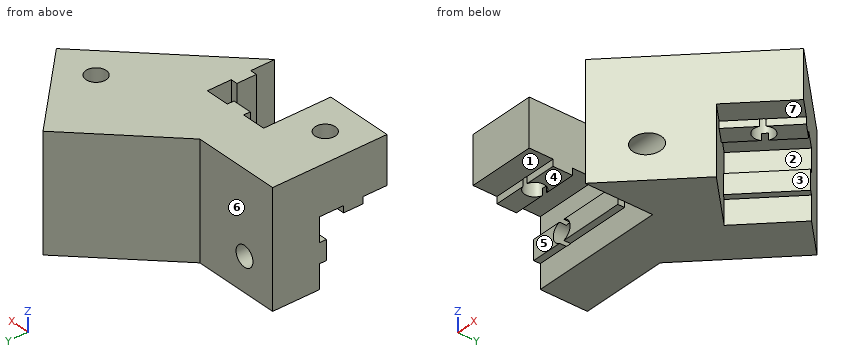
from build123d import *

# Parameters (mm, degrees)
MAIN_DEPTH          = 17
CUT_EXTRUDE1_DEPTH  = 10
SKETCH3_R           = 1.5
CUT_EXTRUDE2_DEPTH  = 18
SKETCH4_W           = 2.9
SKETCH4_H           = 1
SKETCH4_W_2         = 1
SKETCH4_H_2         = 2.9
BOSS_EXTRUDE1_DEPTH = 7
SKETCH5_W           = 15
SKETCH5_H           = 2.9
BOSS_EXTRUDE2_DEPTH = 1
SKETCH6_R           = 1.5
CUT_EXTRUDE3_DEPTH  = 18
BOSS_EXTRUDE3_DEPTH = 10
SKETCH8_R           = 1.5
CUT_EXTRUDE4_DEPTH  = 18
SKETCH9_R           = 1.5
CUT_EXTRUDE5_DEPTH  = 18.67766953


with BuildPart() as part:
    # Sketch1 → Main (new body)
    with BuildSketch(Plane.XY):
        Polygon((-90, -90), (-72.32233047, -72.32233047), (-84.343145751, -60.30151519), (-97.04163056, -73), (-110, -73), (-110, -80), (-90, -80), align=None)
    extrude(amount=MAIN_DEPTH)

    # Sketch2 → Cut-Extrude1 (cut)
    with BuildSketch(Plane(origin=(-72.32233047, -72.32233047, 0), x_dir=(0.707106781, -0.707106781, 0), z_dir=(0.707106781, 0.707106781, 0))):
        Polygon((-3.55, -10), (0, -10), (0, 0), (-10, 0), (-10, -3.55), (-9, -3.55), (-9, -6.45), (-10, -6.45), (-10, -10), (-6.45, -10), (-6.45, -9), (-3.55, -9), align=None)
    extrude(amount=-CUT_EXTRUDE1_DEPTH, mode=Mode.SUBTRACT)

    # Sketch3 → Cut-Extrude2 (cut, through all)
    with BuildSketch(Plane.XY.offset(17)):
        with Locations((-79.393398282, -72.32233047)):
            Circle(SKETCH3_R)
    extrude(amount=-CUT_EXTRUDE2_DEPTH, mode=Mode.SUBTRACT)

    # Sketch4 → Boss-Extrude1 (add)
    with BuildSketch(Plane.XY.offset(10)):
        with Locations((-95, -80.5)):
            Rectangle(SKETCH4_W, SKETCH4_H)
        with Locations((-90.5, -85)):
            Rectangle(SKETCH4_W_2, SKETCH4_H_2)
    extrude(amount=BOSS_EXTRUDE1_DEPTH)

    # Sketch5 → Boss-Extrude2 (add)
    with BuildSketch(Plane.XZ.offset(80)):
        with Locations((-102.5, 5)):
            Rectangle(SKETCH5_W, SKETCH5_H)
    extrude(amount=BOSS_EXTRUDE2_DEPTH)

    # Sketch6 → Cut-Extrude3 (cut, through all)
    with BuildSketch(Plane(origin=(0, -73, 0), x_dir=(1, 0, 0), z_dir=(0, 1, 0))):
        with Locations((-105, -5)):
            Circle(SKETCH6_R)
    extrude(amount=-CUT_EXTRUDE3_DEPTH, mode=Mode.SUBTRACT)

    # Sketch7 → Boss-Extrude3 (add)
    with BuildSketch(Plane.ZY.offset(110)):
        Polygon((17, -80), (17, -90), (10, -90), (10, -86.45), (9, -86.45), (9, -83.55), (10, -83.55), (10, -80), align=None)
    extrude(amount=-BOSS_EXTRUDE3_DEPTH)

    # Sketch8 → Cut-Extrude4 (cut, through all)
    with BuildSketch(Plane.XY.offset(17)):
        with Locations((-105, -85)):
            Circle(SKETCH8_R)
    extrude(amount=-CUT_EXTRUDE4_DEPTH, mode=Mode.SUBTRACT)

    # Sketch9 → Cut-Extrude5 (cut, through all)
    with BuildSketch(Plane.ZY.offset(90)):
        with Locations((5, -85)):
            Circle(SKETCH9_R)
    extrude(amount=-CUT_EXTRUDE5_DEPTH, mode=Mode.SUBTRACT)


solid = part.part
The listing builds one solid part. Answer for the finished solid, in the listing's coordinates (mm). Face numbers are marked on the shaded views. A direction names the side the tool comes from. Coordinates: 2 decimals unless noted, no trailing zeros. Write each loop counter-clockwise with the first axis right and the second up, starting at its lowest first coordinate (ties: lowest second). Pieces come first, ordered by that corner, then holes. Notation, with made-up numbers: M -11,41.5 L -3,41.5 A13 cw -3,49.5 Z; hole C 8,35.25 d4. An arc over 180 degrees is marked long. Put each result on its own line as item: value. Start each with the question number.
1. Consider line 1 (Z direction, x = -85.75, y = -85); line 2 (Y direction, x = -105, z = 15.75); line 3 (Z direction, x = -78, y = -73.25). Determine where each line is inside the solid, lowest interval first. Write a range as from..to.
2. Flat-ended cylindrical pins translate along their axes: P1, Ø4, axis at x = -86, z = 7.5, coming from the -Y side; P2, Ø4, axis at y = -86, z = 6, coming from the -X side; P3, Ø3, axis at y = -84.5, z = 6, coming from the +X side. Find the tip coordinate at first contact, or state that the pin passes through.
3. For a pull along Y with two mould halves and no side action, classify the marked faces 4, 5, 6 and 7 as pulls with the +Y half, pulls with the -Y half, needs draft (parallel to the pull), parting line crosses it, or undercut.
4. A cutting plane is placed at B-B on z = 15.5. Write down the section's boundary in (x, y), then the cut area to 3 significant figures.
5. Which of the six approach directions +Z, -Z, +X, -X, +Y, -Y give full straight-line access (tool end or side, diameter ignored) to the marked faces 1, 2 and 3?
6. A cutting plane is placed at C-C on z = 5. Write down the section's boundary in (x, y), then the cut area to 3 significant figures.
7. A cutting plane is placed at D-D on z = 7.75. Write down the section's boundary in (x, y), then the cut area to 3 significant figures.
8. A cutting plane is placed at A-A on y = -85. Write down the section's boundary in (x, z).
Resolved:
1. line 1: z = 0..3.5, 6.5..17
1. line 2: y = -90..-86.5, -83.5..-73
1. line 3: z = 10..17
2. P1: stops at y = -88
2. P2: stops at x = -90
2. P3: stops at x = -83
3. face 4: needs draft
3. face 5: pulls with the -Y half
3. face 6: pulls with the +Y half
3. face 7: undercut
4. outline: M -110,-90 L -100,-90 L -100,-80 L -96.45,-80 L -96.45,-81 L -93.55,-81 L -93.55,-80 L -90,-80 L -90,-83.55 L -91,-83.55 L -91,-86.45 L -90,-86.45 L -90,-90 L -72.32,-72.32 L -84.34,-60.3 L -97.04,-73 L -110,-73 Z; hole C -105,-85 d3; hole C -79.39,-72.32 d3
4. area: 537 mm2
5. face 1: -Z, -X, -Y
5. face 2: none
5. face 3: -Z, +X
6. outline: M -110,-81 L -106.5,-81 L -106.5,-73 L -110,-73 Z; M -103.5,-81 L -95,-81 L -95,-80 L -90,-80 L -90,-83.5 L -83.5,-83.5 L -79.39,-79.39 L -85.76,-73.03 L -78.69,-65.96 L -84.34,-60.3 L -97.04,-73 L -103.5,-73 Z; M -90,-90 L -86.5,-86.5 L -90,-86.5 Z
6. area: 331 mm2
7. outline: M -110,-80 L -90,-80 L -90,-90 L -79.39,-79.39 L -86.46,-72.32 L -79.39,-65.25 L -84.34,-60.3 L -97.04,-73 L -110,-73 Z
7. area: 345 mm2
8. outline: M -110,9 L -106.5,9 L -106.5,17 L -110,17 Z; M -103.5,9 L -100,9 L -100,17 L -103.5,17 Z; M -91,10 L -90,10 L -90,6.5 L -85,6.5 L -85,17 L -91,17 Z; M -90,0 L -85,0 L -85,3.5 L -90,3.5 Z
